```python
from build123d import *

# Parameters (mm, degrees)
SKETCH_1_W             = 30
SKETCH_1_H             = 40
SKETCH_1_W_2           = 27
SKETCH_1_H_2           = 37
EXTRUDE_1_DEPTH        = 980
SKETCH_3_R             = 1.5
CUT_EXTRUDE_2_DEPTH    = 981.930680527
SKETCH_4_R             = 1.5
CUT_EXTRUDE_3_DEPTH    = 981.930680527
SKETCH_5_R             = 1.5
CUT_EXTRUDE_4_DEPTH    = 981.930680527
CUT_EXTRUDE_6_DEPTH    = 10
SKETCH_9_R             = 3.25
CUT_EXTRUDE_7_DEPTH    = 10
PATTERN_LINEAR_1_COUNT = 4
PATTERN_LINEAR_1_PITCH = 15
SKETCH_10_R            = 2.55
CUT_EXTRUDE_8_DEPTH    = 51
SKETCH_11_R            = 2
CUT_EXTRUDE_9_DEPTH    = 51
SKETCH_12_R            = 2.1
CUT_EXTRUDE_10_DEPTH   = 10
CUT_EXTRUDE_11_DEPTH   = 10


with BuildPart() as part:
    # 草图1 → 凸台-拉伸1 (new body)
    with BuildSketch(Plane.XY):
        Rectangle(SKETCH_1_W, SKETCH_1_H)
        Rectangle(SKETCH_1_W_2, SKETCH_1_H_2, mode=Mode.SUBTRACT)
    extrude(amount=EXTRUDE_1_DEPTH)

    # 草图3 → 切除-拉伸2 (cut, through all)
    with BuildSketch(Plane(origin=(0, 20, 0), x_dir=(-1, 0, 0), z_dir=(0, -1, 0))):
        with Locations(Location((5, -10, 0), (0, 0, 180))):
            Circle(SKETCH_3_R)
        with Locations(Location((-5, -10, 0), (0, 0, 270))):
            Circle(SKETCH_3_R)
        with Locations(Location((-5, -970, 0), (0, 0, 180))):
            Circle(SKETCH_3_R)
        with Locations(Location((5, -970, 0), (0, 0, 270))):
            Circle(SKETCH_3_R)
    extrude(amount=CUT_EXTRUDE_2_DEPTH, mode=Mode.SUBTRACT)

    # 草图4 → 切除-拉伸3 (cut, through all)
    with BuildSketch(Plane(origin=(0, 20, 0), x_dir=(-1, 0, 0), z_dir=(0, -1, 0))):
        with Locations(Location((-8.27006126, -772.5, 0), (0, 0, 180))):
            Circle(SKETCH_4_R)
        with Locations(Location((6.72993874, -772.5, 0), (0, 0, 270))):
            Circle(SKETCH_4_R)
        with Locations(Location((6.72993874, -787.5, 0), (0, 0, 180))):
            Circle(SKETCH_4_R)
        with Locations(Location((-8.27006126, -787.5, 0), (0, 0, 270))):
            Circle(SKETCH_4_R)
    cut_extrude_3 = extrude(amount=CUT_EXTRUDE_3_DEPTH, mode=Mode.SUBTRACT)

    # 草图5 → 切除-拉伸4 (cut, through all)
    with BuildSketch(Plane(origin=(0, 20, 0), x_dir=(-1, 0, 0), z_dir=(0, -1, 0))):
        with Locations(Location((0, -140, 0), (0, 0, 180))):
            Circle(SKETCH_5_R)
        with Locations(Location((0, -160, 0), (0, 0, 180))):
            Circle(SKETCH_5_R)
        with Locations(Location((0, -300, 0), (0, 0, 180))):
            Circle(SKETCH_5_R)
        with Locations(Location((0, -320, 0), (0, 0, 180))):
            Circle(SKETCH_5_R)
        with Locations(Location((0, -480, 0), (0, 0, 180))):
            Circle(SKETCH_5_R)
        with Locations(Location((0, -460, 0), (0, 0, 180))):
            Circle(SKETCH_5_R)
    extrude(amount=CUT_EXTRUDE_4_DEPTH, mode=Mode.SUBTRACT)

    # 草图8 → 切除-拉伸6 (cut)
    with BuildSketch(Plane.XZ.offset(20)):
        with BuildLine():
            Line((7.5, 160), (7.5, 140))
            ThreePointArc((7.5, 140), (0, 132.5), (-7.5, 140))
            Line((-7.5, 140), (-7.5, 160))
            ThreePointArc((-7.5, 160), (0, 167.5), (7.5, 160))
        make_face()
        with BuildLine():
            Line((7.5, 480), (7.5, 460))
            ThreePointArc((7.5, 460), (0, 452.5), (-7.5, 460))
            Line((-7.5, 460), (-7.5, 480))
            ThreePointArc((-7.5, 480), (0, 487.5), (7.5, 480))
        make_face()
        with BuildLine():
            Line((7.5, 320), (7.5, 300))
            ThreePointArc((7.5, 300), (0, 292.5), (-7.5, 300))
            Line((-7.5, 300), (-7.5, 320))
            ThreePointArc((-7.5, 320), (0, 327.5), (7.5, 320))
        make_face()
    extrude(amount=-CUT_EXTRUDE_6_DEPTH, mode=Mode.SUBTRACT)

    # 草图9 → 切除-拉伸7 (cut)
    with BuildSketch(Plane.XZ.offset(20)):
        with Locations(Location((-6.72993874, 787.5, 0), (0, 0, 270))):
            Circle(SKETCH_9_R)
        with Locations(Location((-6.72993874, 772.5, 0), (0, 0, 270))):
            Circle(SKETCH_9_R)
        with Locations(Location((8.27006126, 772.5, 0), (0, 0, 270))):
            Circle(SKETCH_9_R)
        with Locations(Location((8.27006126, 787.5, 0), (0, 0, 270))):
            Circle(SKETCH_9_R)
    cut_extrude_7 = extrude(amount=-CUT_EXTRUDE_7_DEPTH, mode=Mode.SUBTRACT)

    # 阵列(线性)1: 切除-拉伸3, 切除-拉伸7 ×4
    with Locations(*[(0, 0, -i * PATTERN_LINEAR_1_PITCH) for i in range(1, PATTERN_LINEAR_1_COUNT)]):
        add(cut_extrude_3, mode=Mode.SUBTRACT)
        add(cut_extrude_7, mode=Mode.SUBTRACT)

    # 草图10 → 切除-拉伸8 (cut)
    with BuildSketch(Plane.ZY.offset(15)):
        with Locations((646, 12)):
            Circle(SKETCH_10_R)
        with Locations((670, 12)):
            Circle(SKETCH_10_R)
        with Locations((646, -12)):
            Circle(SKETCH_10_R)
        with Locations((670, -12)):
            Circle(SKETCH_10_R)
    extrude(amount=-CUT_EXTRUDE_8_DEPTH, mode=Mode.SUBTRACT)

    # 草图11 → 切除-拉伸9 (cut)
    with BuildSketch(Plane.ZY.offset(15)):
        with Locations((725, 10.625214933)):
            Circle(SKETCH_11_R)
        with Locations((725, -9.374785067)):
            Circle(SKETCH_11_R)
        with Locations((735, 10.625214933)):
            Circle(SKETCH_11_R)
        with Locations((735, -9.374785067)):
            Circle(SKETCH_11_R)
        with Locations((745, 10.625214933)):
            Circle(SKETCH_11_R)
        with Locations((745, -9.374785067)):
            Circle(SKETCH_11_R)
        with Locations((755, 10.625214933)):
            Circle(SKETCH_11_R)
        with Locations((755, -9.374785067)):
            Circle(SKETCH_11_R)
        with Locations((765, 10.625214933)):
            Circle(SKETCH_11_R)
        with Locations((765, -9.374785067)):
            Circle(SKETCH_11_R)
        with Locations((775, 10.625214933)):
            Circle(SKETCH_11_R)
        with Locations((775, -9.374785067)):
            Circle(SKETCH_11_R)
        with Locations((785, 10.625214933)):
            Circle(SKETCH_11_R)
        with Locations((785, -9.374785067)):
            Circle(SKETCH_11_R)
        with Locations((795, 10.625214933)):
            Circle(SKETCH_11_R)
        with Locations((795, -9.374785067)):
            Circle(SKETCH_11_R)
        with Locations((805, 10.625214933)):
            Circle(SKETCH_11_R)
        with Locations((805, -9.374785067)):
            Circle(SKETCH_11_R)
        with Locations((815, 10.625214933)):
            Circle(SKETCH_11_R)
        with Locations((815, -9.374785067)):
            Circle(SKETCH_11_R)
        with Locations((825, 10.625214933)):
            Circle(SKETCH_11_R)
        with Locations((825, -9.374785067)):
            Circle(SKETCH_11_R)
        with Locations((835, 10.625214933)):
            Circle(SKETCH_11_R)
        with Locations((835, -9.374785067)):
            Circle(SKETCH_11_R)
    extrude(amount=-CUT_EXTRUDE_9_DEPTH, mode=Mode.SUBTRACT)

    # 草图12 → 切除-拉伸10 (cut)
    with BuildSketch(Plane(origin=(0, 20, 0), x_dir=(1, 0, 0), z_dir=(0, 1, 0))):
        with Locations(Location((-7, -45, 0), (0, 0, 270))):
            Circle(SKETCH_12_R)
        with Locations(Location((-7, -57, 0), (0, 0, 270))):
            Circle(SKETCH_12_R)
        with Locations((7, -57)):
            Circle(SKETCH_12_R)
        with Locations((7, -45)):
            Circle(SKETCH_12_R)
    extrude(amount=-CUT_EXTRUDE_10_DEPTH, mode=Mode.SUBTRACT)

    # 草图13 → 切除-拉伸11 (cut)
    with BuildSketch(Plane.XZ.offset(20)):
        with BuildLine():
            Line((-9, 27.5), (-9, 72.5))
            ThreePointArc((-9, 72.5), (0, 81.5), (9, 72.5))
            Line((9, 72.5), (9, 27.5))
            ThreePointArc((9, 27.5), (0, 18.5), (-9, 27.5))
        make_face()
    extrude(amount=-CUT_EXTRUDE_11_DEPTH, mode=Mode.SUBTRACT)


solid = part.part
```
CAD build for the part. Positions are in the model's coordinates, mm. A direction names the side the tool comes from. Coordinates: 2 decimals unless noted, no trailing zeros. Order: outer loops, then holes, each group sorted by start corner. A loop starts at its lowest first (then second) coordinate and runs counter-clockwise, first axis right, second up. Notation, with made-up numbers: (35, -13) - (45, -13) arc R26 ccw to (45, 22) - close; hole circle Ø11 at (43, 60). An arc over 180 degrees is marked (long way). Use a Markdown table: item, result. Add a question column.
(1) Drill centre lines: line 1 along X through (y, z) = (18.9, 10); line 2 along X through (y, z) = (3.5, 936.5); line 3 along Y through (x, z) = (10.25, 277). Where is each one in solid material? Low to high. Write a range as [from, to].
(2) Pull direction Y, two halves, no side cores. Call faces 3 (the face through (-14.5, 0.1, 0)), 4 (the face through (0, 20, 483)), 5 (the face through (0, 18.5, 483)), 6 (the face through (0, -18.5, 592)): +Y half, -Y half, draft (parallel to the pull), parting line (faces both ways), or undercut.
(3) Saw through at A-A (z = 228). Give the cut face in (x, y), then the cut area to 3 significant figures.
(4) Which spindle directions (+Z, -Z, +X, -X, +Y, -Y) get a long thin tool onto all of the face, cutting with end or side? Do faces 1 (the face through (-14.5, 0.1, 980)), 2 (the face through (-13.5, 0, 483)). Say none if no direction does.
Solved:
| question | item | result |
|---|---|---|
| 1 | line 1 | x = [-15, -6.5], [-3.5, 3.5], [6.5, 15] |
| 1 | line 2 | x = [-15, -13.5], [13.5, 15] |
| 1 | line 3 | y = [-20, -18.5], [18.5, 20] |
| 2 | face 3 | draft |
| 2 | face 4 | +Y half |
| 2 | face 5 | undercut |
| 2 | face 6 | undercut |
| 3 | outline | (-15, -20) - (15, -20) - (15, 20) - (-15, 20) - close; hole (-13.5, -18.5) - (13.5, -18.5) - (13.5, 18.5) - (-13.5, 18.5) - close |
| 3 | area | 201 mm² |
| 4 | face 1 | +Z, +X, -X, +Y, -Y |
| 4 | face 2 | +Z, -Z |
